```python
from build123d import *

# Parameters (mm, degrees)
F0_W            = 59
F0_H            = 59
F3_DEPTH        = 15
F1_W            = 53
F1_H            = 53
F4_DEPTH        = 12
F5_R            = 2
F7_R            = 5
F8_DEPTH        = 6
F10_D           = 4.4
F10_CBORE_D     = 8.25
F10_CBORE_DEPTH = 4
F11_D           = 4.4
F11_CBORE_D     = 8.25
F11_CBORE_DEPTH = 4
F12_D           = 4.4
F12_CBORE_D     = 8.25
F12_CBORE_DEPTH = 4
F13_D           = 4.4
F13_CBORE_D     = 8.25
F13_CBORE_DEPTH = 4
F14_DEPTH       = 30


with BuildPart() as f3:
    # F0 (on Front) → F3 (new body)
    with BuildSketch(Plane.XZ):
        Rectangle(F0_W, F0_H)
    extrude(amount=F3_DEPTH)

    # F1 (on Front) → F4 (cut)
    with BuildSketch(Plane.XZ):
        Rectangle(F1_W, F1_H)
    extrude(amount=F4_DEPTH, mode=Mode.SUBTRACT)

    # F5
    f5_edges = [f3.edges().sort_by_distance(p)[0] for p in [
        (0, -15, 29.5),
        (-29.5, -15, 0),
        (0, -15, -29.5),
        (29.5, -15, 0),
    ]]
    fillet(f5_edges, radius=F5_R)

    # F7 (on offset) → F8 (join)
    with BuildSketch(Plane.XZ.offset(15)):
        with Locations((19.5, 19.5)):
            Circle(F7_R)
        with Locations((-19.5, 19.5)):
            Circle(F7_R)
        with Locations((19.5, -19.5)):
            Circle(F7_R)
        with Locations((-19.5, -19.5)):
            Circle(F7_R)
    extrude(amount=-F8_DEPTH)

    # F10 (through all)
    with Locations(Plane.XZ.offset(15)):
        with Locations((-19.5, 19.5)):
            CounterBoreHole(F10_D / 2, F10_CBORE_D / 2, F10_CBORE_DEPTH)

    # F11 (through all)
    with Locations(Plane.XZ.offset(15)):
        with Locations((-19.5, -19.5)):
            CounterBoreHole(F11_D / 2, F11_CBORE_D / 2, F11_CBORE_DEPTH)

    # F12 (through all)
    with Locations(Plane.XZ.offset(15)):
        with Locations((19.5, -19.5)):
            CounterBoreHole(F12_D / 2, F12_CBORE_D / 2, F12_CBORE_DEPTH)

    # F13 (through all)
    with Locations(Plane.XZ.offset(15)):
        with Locations((19.5, 19.5)):
            CounterBoreHole(F13_D / 2, F13_CBORE_D / 2, F13_CBORE_DEPTH)

    # F2 (on Top) → F14 (cut, symmetric)
    with BuildSketch(Plane.XY):
        with BuildLine():
            Line((8.1, 2.8), (-8.1, 2.8))
            ThreePointArc((-8.1, 2.8), (-8.8071067812, 2.5071067812), (-9.1, 1.8))
            Line((-9.1, 1.8), (-9.1, -1.8))
            ThreePointArc((-9.1, -1.8), (-8.8071067812, -2.5071067812), (-8.1, -2.8))
            Line((-8.1, -2.8), (8.1, -2.8))
            ThreePointArc((8.1, -2.8), (8.8071067812, -2.5071067812), (9.1, -1.8))
            Line((9.1, -1.8), (9.1, 1.8))
            ThreePointArc((9.1, 1.8), (8.8071067812, 2.5071067812), (8.1, 2.8))
        make_face()
    extrude(amount=F14_DEPTH, both=True, mode=Mode.SUBTRACT)


solid = f3.part
```
Design review of the part built by this model. Coordinates are the model's own, in mm. A direction names the side the tool comes from. Coordinates: 2 decimals unless noted, no trailing zeros. Write each loop counter-clockwise with the first axis right and the second up, starting at its lowest first coordinate (ties: lowest second). Pieces come first, ordered by that corner, then holes. Notation, with made-up numbers: M 28,87 L 76,87 A27 ccw 76,117 Z; hole C 42,16.5 d2. An arc over 180 degrees is marked long. Answer as a JSON object with one key per item and string values.
Item 1: Machinability: for faces 4 (the flat face through (0, -2.8, -28)), 5 (the flat face through (21, -9, 17)), 6 (the cylindrical face through (-22.54, -13.03, -16.71)), which of the approach directions +Z, -Z, +X, -X, +Y, -Y give a long, thin tool a straight path to every point of the face, cutting with its end or side? Answer none if there is none.
Outcome:
{"face 4": "+Z, -Z, +Y", "face 5": "+Y", "face 6": "-Y"}
Item 2: Insertion check: pin 1 Ø2.5 at (x, z) = (19.5, 19.5) entering from -Y; pin 2 Ø3.5 at (x, z) = (-3, -28.5) entering from +Y; pin 3 Ø5 at (x, z) = (-22, 17) entering from +Y; pin 4 Ø5.5 at (x, z) = (-19.5, 19.5) entering from -Y. Each pin has a flat end and moves straight along its axis. Give the tip position at first contact, or say it passes through.
Outcome:
{"pin 1": "through", "pin 2": "y = -2.8", "pin 3": "y = -9", "pin 4": "y = -11"}
Item 3: Wall thickness on probe 1 along Z at (x, y) = (19.5, -10.3); probe 2 along Z at (x, y) = (-19.5, -12.55) (3 decimals); probe 3 along Z at (x, y) = (-2, -4.25): over which ranges is each line inside the solid? List them lowest first.
Outcome:
{"probe 1": "-29.5 to -26.5, -24.5 to -21.7, -17.3 to -14.5, 14.5 to 17.3, 21.7 to 24.5, 26.5 to 29.5", "probe 2": "-29.5 to -23.625, -15.375 to 15.375, 23.625 to 29.5", "probe 3": "-29.5 to -26.5, 26.5 to 29.5"}
Item 4: Add section B-B, the plane y = -4.25. Give the boundary of the cut face in (x, z).
Outcome:
{"outline": "M -29.5,-29.5 L 29.5,-29.5 L 29.5,29.5 L -29.5,29.5 Z; hole M -26.5,-26.5 L 26.5,-26.5 L 26.5,26.5 L -26.5,26.5 Z"}
Item 5: Add section D-D, the plane z = -6. Give the boundary of the cut face in (x, y).
Outcome:
{"outline": "M -29.5,-13 A2 ccw -27.5,-15 L 27.5,-15 A2 ccw 29.5,-13 L 29.5,0 L 26.5,0 L 26.5,-12 L -26.5,-12 L -26.5,0 L -29.5,0 Z"}
Item 6: Draft analysis for pull direction X (two halves, no side actions). For faces 1 (the flat face through (-29.5, -6, 0)), 2 (the cylindrical face through (17.468, -9.986, 18.657)), 3 (the flat face through (0, -6, 29.5)), state which applies: pulls with the +X half, pulls with the -X half, needs draft (parallel to the pull), parting line crosses it, or undercut.
Outcome:
{"face 1": "pulls with the -X half", "face 2": "undercut", "face 3": "needs draft"}
Item 7: Add section A-A, the plane z = 19.5. State how many separate pieces and enclosed holes the cut face has, and give its area (3 significant figures).
Outcome:
{"separate pieces": "3", "enclosed holes": "0", "area": "224 mm²"}
